Geometry: final body of the model. Coordinates: model frame, mm. Face numbers are marked on the shaded views. A direction names the side the tool comes from. Give positions to 0.01 mm unless a question says otherwise; leave off trailing zeros. Write each loop counter-clockwise with the first axis right and the second up, starting at its lowest first coordinate (ties: lowest second). Pieces come first, ordered by that corner, then holes. Notation, with made-up numbers: M 48,36.25 L 64,36.25 A31 cw 64,74.25 Z; hole C 20,15 d3. An arc over 180 degrees is marked long. Use a Markdown table: item, result. Add a question column.
1) Section C-C on z = -20. Return the cut outline in (x, y).
2) Set-up query: the marked faces 1 and 2. Return all of +Z, -Z, +X, -X, +Y, -Y with unobstructed straight access to the full face (end or side cutting, diameter ignored); none if empty.
3) Section A-A on x = -23. Return the cut outline in (y, z).
4) Pin query (flat end, axial travel): pin 1 (1.5 mm diameter, centred on y = -3.5, z = -4.5, fed in from +X); pin 2 (8 mm diameter, centred on y = 2, z = -6.5, fed in from -X); pin 3 (19 mm diameter, centred on x = -30, y = 20.5, fed in from -Z). Return the tip coordinate at first contact, or that it passes through.
5) Section D-D on x = 55. Return the cut outline in (y, z), then the cut area to 3 significant figures.
6) Section B-B on y = 27. Return the cut outline in (x, z), then the cut area to 3 significant figures.
7) Line query: line 1 (Y direction, x = 16, z = 18); line 2 (Y direction, x = -46, z = 1.5); line 3 (Z direction, x = -62, y = 25.5). Output: solid intervals per line, ascending.
```python
from build123d import *

# Parameters (mm, degrees)
SKETCH1_W                    = 139
SKETCH1_H                    = 50
BASE_FLANGE1_DEPTH           = 8
EDGE_FLANGE1_STRIP_W         = 48
EDGE_FLANGE1_STRIP_H         = 8
EDGE_FLANGE1_STRIP_CUT_DEPTH = 139
EDGE_FLANGE1_DEPTH           = 139
CHAMFER1_SIZE                = 43
CHAMFER1_SIZE2               = 30.108924143
MIRROR3_START                = 46.606691224
MIRROR3_OUTLINE_W            = 55
MIRROR3_OUTLINE_H            = 41
MIRROR3_DEPTH                = 24.663786763


# Read off the part's stored shape, not the designer's step: Mirror3
# Sheet-metal steps are written as plain solids
with BuildPart() as part:
    # Sketch1 → Base-Flange1 (new body)
    with BuildSketch(Plane(origin=(0, 0, 0), x_dir=(1, 0, 0), z_dir=(0, 1, 0))):
        Rectangle(SKETCH1_W, SKETCH1_H)
    extrude(amount=-BASE_FLANGE1_DEPTH)

    # Edge-Flange1 strip (across the edge) → Edge-Flange1 strip cut (cut)
    with BuildSketch(Plane(origin=(-69.5, 0, 25), x_dir=(0, 0, -1), z_dir=(1, 0, 0))):
        with Locations((-8, -4)):
            Rectangle(EDGE_FLANGE1_STRIP_W, EDGE_FLANGE1_STRIP_H)
    extrude(amount=EDGE_FLANGE1_STRIP_CUT_DEPTH, mode=Mode.SUBTRACT)

    # Edge-Flange1 section (across the edge) → Edge-Flange1 (add)
    with BuildSketch(Plane(origin=(-69.5, 0, 25), x_dir=(0, 0, -1), z_dir=(1, 0, 0))):
        with BuildLine():
            Line((0, 8), (0, 32))
            Line((0, 32), (8, 32))
            Line((8, 32), (8, 8))
            ThreePointArc((8, 8), (10.343145751, 2.343145751), (16, 0))
            Line((16, 0), (16, -8))
            ThreePointArc((16, -8), (4.686291501, -3.313708499), (0, 8))
        make_face()
    extrude(amount=EDGE_FLANGE1_DEPTH)

    # Chamfer1
    chamfer1_edges = [part.edges().sort_by_distance(p)[0] for p in [
        (-69.5, -4, -25),
    ]]
    chamfer1_side = [part.faces().sort_by_distance(p)[0] for p in [
        (-69.5, -0.640312424, -8),
    ]]
    chamfer(chamfer1_edges, length=CHAMFER1_SIZE, length2=CHAMFER1_SIZE2, reference=chamfer1_side[0])

    # Mirror3 outline → Mirror3 (cut)
    with BuildSketch(Plane(origin=(0, 0, 0), x_dir=(0.5735764363510512, 0, 0.8191520442889882), z_dir=(0.8191520442889882, 0, -0.5735764363510512)).offset(MIRROR3_START)):
        with Locations((28.5, -12.5)):
            Rectangle(MIRROR3_OUTLINE_W, MIRROR3_OUTLINE_H)
    extrude(amount=MIRROR3_DEPTH, mode=Mode.SUBTRACT)


solid = part.part
```
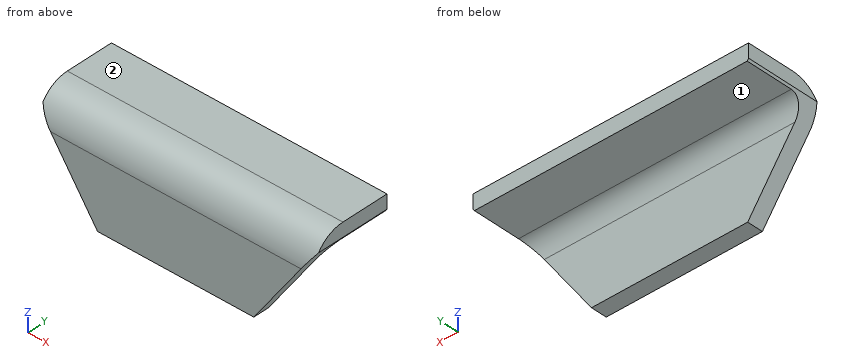
Found:
| question | item | result |
|---|---|---|
| 1 | outline | M -42.89,-8 L 42.89,-8 L 42.89,0 L -42.89,0 Z |
| 2 | face 1 | -Z, +X, -X, +Y |
| 2 | face 2 | +Z, +X, -X, +Y, -Y |
| 3 | outline | M -8,-25 L 0,-25 L 0,9 A8 cw 8,17 L 32,17 L 32,25 L 8,25 A16 ccw -8,9 Z |
| 4 | pin 1 | x = 54.27 |
| 4 | pin 2 | x = -54.77 |
| 4 | pin 3 | z = 17 |
| 5 | outline | M -8,-2.71 L 0,-2.71 L 0,9 A8 cw 8,17 L 32,17 L 32,25 L 8,25 A16 ccw -8,9 Z |
| 5 | area | 436 mm² |
| 6 | outline | M -69.5,18 L -68.8,17 L 68.8,17 L 69.5,18 L 69.5,25 L -69.5,25 Z |
| 6 | area | 1,110 mm² |
| 7 | line 1 | -5.23 to 32 |
| 7 | line 2 | -8 to 0 |
| 7 | line 3 | 17 to 25 |
